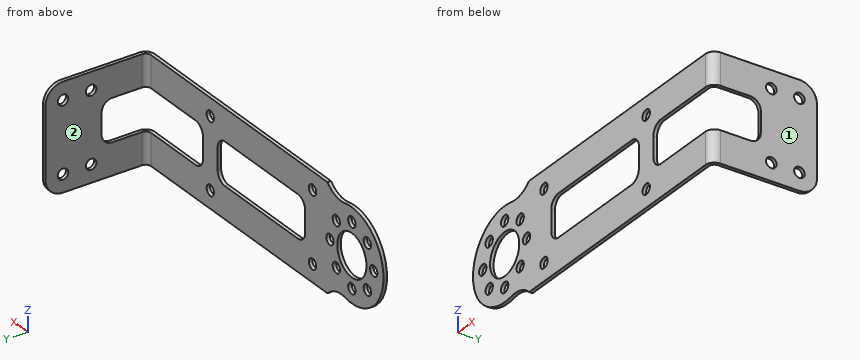
```python
from build123d import *

# Parameters (mm, degrees)
BASE_FLANGE1_DEPTH           = 1
EDGE_FLANGE1_STRIP_W         = 7
EDGE_FLANGE1_STRIP_H         = 1
EDGE_FLANGE1_STRIP_CUT_DEPTH = 30
EDGE_FLANGE1_DEPTH           = 30
FILLET1_R                    = 5
UNFOLD1_OUTLINE_W            = 3.141592654
UNFOLD1_OUTLINE_H            = 30
UNFOLD1_DEPTH                = 29
UNFOLD1_START                = -1
UNFOLD1_2_DEPTH              = 1
SKETCH10_R                   = 6
SKETCH10_R_2                 = 1.5
SKETCH10_W                   = 36
SKETCH10_H                   = 12
CUT_EXTRUDE1_DEPTH           = 10
FILLET2_R                    = 3
FOLD1_START                  = 84.74315
FOLD1_OUTLINE_W              = 1
FOLD1_OUTLINE_H              = 30
FOLD1_DEPTH                  = 28.398442654
FOLD1_START_2                = 82.5
FOLD1_2_OUTLINE_R            = 1.5
FOLD1_2_DEPTH                = 2.5
FOLD1_START_3                = -16
FOLD1_3_DEPTH                = 31


with BuildPart() as part:
    # Base-Flange1: sheet metal written as solids
    # Sketch1 → Base-Flange1 (new body)
    with BuildSketch(Plane(origin=(0, 0, 0), x_dir=(1, 0, 0), z_dir=(0, 1, 0))):
        with BuildLine():
            Line((10, -15), (85, -15))
            Line((85, -15), (85, 15))
            Line((85, 15), (10, 15))
            ThreePointArc((10, 15), (6.607674197, 12.919380101), (2.632597571, 12.730649238))
            ThreePointArc((2.632597571, 12.730649238), (-13, 0), (2.632597571, -12.730649238))
            ThreePointArc((2.632597571, -12.730649238), (6.607674197, -12.919380101), (10, -15))
        make_face()
    extrude(amount=-BASE_FLANGE1_DEPTH)

    # Edge-Flange1: sheet metal written as solids
    # Edge-Flange1 strip (on a plane across the edge) → Edge-Flange1 strip cut (cut)
    with BuildSketch(Plane(origin=(85, 0, 15), x_dir=(-1, 0, 0), z_dir=(0, 0, -1))):
        with Locations((-1, -0.5)):
            Rectangle(EDGE_FLANGE1_STRIP_W, EDGE_FLANGE1_STRIP_H)
    extrude(amount=EDGE_FLANGE1_STRIP_CUT_DEPTH, mode=Mode.SUBTRACT)

    # Edge-Flange1 section (on a plane across the edge) → Edge-Flange1 (add)
    with BuildSketch(Plane(origin=(85, 0, 15), x_dir=(-1, 0, 0), z_dir=(0, 0, -1))):
        with BuildLine():
            Line((0, 1.5), (0, 29))
            Line((0, 29), (1, 29))
            Line((1, 29), (1, 1.5))
            ThreePointArc((1, 1.5), (1.439339828, 0.439339828), (2.5, 0))
            Line((2.5, 0), (2.5, -1))
            ThreePointArc((2.5, -1), (0.732233047, -0.267766953), (0, 1.5))
        make_face()
    extrude(amount=EDGE_FLANGE1_DEPTH)

    # Fillet1
    fillet1_edges = [part.edges().sort_by_distance(p)[0] for p in [
        (84.5, 29, 15),
        (84.5, 29, -15),
    ]]
    fillet(fillet1_edges, radius=FILLET1_R)

    # Unfold1: read off the stored shape, not the designer's step
    # Unfold1 outline → Unfold1 (cut)
    with BuildSketch(Plane(origin=(0, 0, 0), x_dir=(1, 0, 0), z_dir=(0, 1, 0))):
        with Locations((84.070796327, 0)):
            Rectangle(UNFOLD1_OUTLINE_W, UNFOLD1_OUTLINE_H)
    extrude(amount=UNFOLD1_DEPTH, mode=Mode.SUBTRACT)

    # Unfold1 2 outline → Unfold1 2 (add)
    with BuildSketch(Plane(origin=(0, 0, 0), x_dir=(1, 0, 0), z_dir=(0, 1, 0)).offset(UNFOLD1_START)):
        with BuildLine():
            Line((108.141592654, 15), (82.5, 15))
            Line((82.5, 15), (82.5, -15))
            Line((82.5, -15), (108.141592654, -15))
            ThreePointArc((108.141592654, -15), (111.67712656, -13.535533906), (113.141592654, -10))
            Line((113.141592654, -10), (113.141592654, 10))
            ThreePointArc((113.141592654, 10), (111.67712656, 13.535533906), (108.141592654, 15))
        make_face()
    extrude(amount=UNFOLD1_2_DEPTH)

    # Sketch10 → Cut-Extrude1 (cut)
    with BuildSketch(Plane(origin=(0, 0, 0), x_dir=(1, 0, 0), z_dir=(0, 1, 0))):
        with Locations(Location((0, 0, 0), (0, 0, 270))):
            Circle(SKETCH10_R)
        with Locations(Location((0, 9, 0), (0, 0, 270))):
            Circle(SKETCH10_R_2)
        with Locations(Location((6.363961031, 6.363961031, 0), (0, 0, 270))):
            Circle(SKETCH10_R_2)
        with Locations(Location((9, 0, 0), (0, 0, 270))):
            Circle(SKETCH10_R_2)
        with Locations(Location((6.363961031, -6.363961031, 0), (0, 0, 270))):
            Circle(SKETCH10_R_2)
        with Locations(Location((0, -9, 0), (0, 0, 270))):
            Circle(SKETCH10_R_2)
        with Locations(Location((-6.363961031, -6.363961031, 0), (0, 0, 270))):
            Circle(SKETCH10_R_2)
        with Locations(Location((-9, 0, 0), (0, 0, 270))):
            Circle(SKETCH10_R_2)
        with Locations(Location((-6.363961031, 6.363961031, 0), (0, 0, 270))):
            Circle(SKETCH10_R_2)
        with Locations(Location((16.141592654, 10, 0), (0, 0, 270))):
            Circle(SKETCH10_R_2)
        with Locations(Location((16.141592654, -10, 0), (0, 0, 270))):
            Circle(SKETCH10_R_2)
        with Locations(Location((58.141592654, 10, 0), (0, 0, 270))):
            Circle(SKETCH10_R_2)
        with Locations(Location((58.141592654, -10, 0), (0, 0, 270))):
            Circle(SKETCH10_R_2)
        with Locations(Location((100.141592654, 10, 0), (0, 0, 270))):
            Circle(SKETCH10_R_2)
        with Locations(Location((108.141592654, 10, 0), (0, 0, 270))):
            Circle(SKETCH10_R_2)
        with Locations(Location((100.141592654, -10, 0), (0, 0, 270))):
            Circle(SKETCH10_R_2)
        with Locations(Location((108.141592654, -10, 0), (0, 0, 270))):
            Circle(SKETCH10_R_2)
        with Locations((37.141592654, 0)):
            Rectangle(SKETCH10_W, SKETCH10_H)
        with Locations((79.141592654, 0)):
            Rectangle(SKETCH10_W, SKETCH10_H)
    extrude(amount=-CUT_EXTRUDE1_DEPTH, mode=Mode.SUBTRACT)

    # Fillet2
    fillet2_edges = [part.edges().sort_by_distance(p)[0] for p in [
        (97.141592654, -0.5, -6),
        (97.141592654, -0.5, 6),
        (61.141592654, -0.5, 6),
        (61.141592654, -0.5, -6),
        (55.141592654, -0.5, -6),
        (55.141592654, -0.5, 6),
        (19.141592654, -0.5, 6),
        (19.141592654, -0.5, -6),
    ]]
    fillet(fillet2_edges, radius=FILLET2_R)

    # Fold1: read off the stored shape, not the designer's step
    # Fold1 outline → Fold1 (cut)
    with BuildSketch(Plane.YZ.offset(FOLD1_START)):
        with Locations((-0.5, 0)):
            Rectangle(FOLD1_OUTLINE_W, FOLD1_OUTLINE_H)
    extrude(amount=FOLD1_DEPTH, mode=Mode.SUBTRACT)

    # Fold1 2 outline → Fold1 2 (add)
    with BuildSketch(Plane.YZ.offset(FOLD1_START_2)):
        with BuildLine():
            Line((10, -6), (0, -6))
            Line((0, -6), (0, -15))
            Line((0, -15), (24, -15))
            ThreePointArc((24, -15), (27.535533906, -13.535533906), (29, -10))
            Line((29, -10), (29, 10))
            ThreePointArc((29, 10), (27.535533906, 13.535533906), (24, 15))
            Line((24, 15), (0, 15))
            Line((0, 15), (0, 6))
            Line((0, 6), (10, 6))
            ThreePointArc((10, 6), (12.121320344, 5.121320344), (13, 3))
            Line((13, 3), (13, -3))
            ThreePointArc((13, -3), (12.121320344, -5.121320344), (10, -6))
        make_face()
        with Locations((16, -10)):
            Circle(FOLD1_2_OUTLINE_R, mode=Mode.SUBTRACT)
        with Locations((24, -10)):
            Circle(FOLD1_2_OUTLINE_R, mode=Mode.SUBTRACT)
        with Locations((16, 10)):
            Circle(FOLD1_2_OUTLINE_R, mode=Mode.SUBTRACT)
        with Locations((24, 10)):
            Circle(FOLD1_2_OUTLINE_R, mode=Mode.SUBTRACT)
    extrude(amount=FOLD1_2_DEPTH)

    # Fold1 3 outline → Fold1 3 (cut)
    with BuildSketch(Plane.XY.offset(FOLD1_START_3)):
        with BuildLine():
            Line((84, 29), (82.5, 29))
            Line((82.5, 29), (82.5, 0))
            ThreePointArc((82.5, 0), (83.560660172, 0.439339828), (84, 1.5))
            Line((84, 1.5), (84, 29))
        make_face()
        with BuildLine():
            Line((85, 0), (85, 1.5))
            ThreePointArc((85, 1.5), (84.267766953, -0.267766953), (82.5, -1))
            Line((82.5, -1), (84.74315, -1))
            Line((84.74315, -1), (84.74315, 0))
            Line((84.74315, 0), (85, 0))
        make_face()
    extrude(amount=FOLD1_3_DEPTH, mode=Mode.SUBTRACT)


solid = part.part
```
For this review, take the finished solid that the model builds, in its own axes (mm). Face numbers are marked on the shaded views. A direction names the side the tool comes from. Round coordinates to 2 decimals unless told otherwise and drop trailing zeros. Order: outer loops, then holes, each group sorted by start corner. A loop starts at its lowest first (then second) coordinate and runs counter-clockwise, first axis right, second up. Notation, with made-up numbers: (85, 77.5) -> (139, 77.5) arc R21 cw to (139, 89.5) -> close; hole circle Ø8 at (14.25, 70). An arc over 180 degrees is marked (long way). Use a Markdown table: item, result.
Item 1: Take a section at A-A (y = 8.5). State the section outline as (x, z) points, plus the area to 3 significant figures.
Resolved:
| item | result |
|---|---|
| outline | (84, -15) -> (85, -15) -> (85, -6) -> (84, -6) -> close; (84, 6) -> (85, 6) -> (85, 15) -> (84, 15) -> close |
| area | 18.0 mm² |
Item 2: Take a section at B-B (z = 0). State the section outline as (x, y) points, plus the area to 3 significant figures.
Resolved:
| item | result |
|---|---|
| outline | (-13, -1) -> (-10.5, -1) -> (-10.5, 0) -> (-13, 0) -> close; (-7.5, -1) -> (-6, -1) -> (-6, 0) -> (-7.5, 0) -> close; (6, -1) -> (7.5, -1) -> (7.5, 0) -> (6, 0) -> close; (10.5, -1) -> (19.14, -1) -> (19.14, 0) -> (10.5, 0) -> close; (55.14, -1) -> (61.14, -1) -> (61.14, 0) -> (55.14, 0) -> close; (84, 13) -> (85, 13) -> (85, 29) -> (84, 29) -> close |
| area | 36.1 mm² |
Item 3: For pin 1 (4 mm diameter, centred on x = 58.14, z = 10, fed in from +Y); pin 2 (1.1 mm diameter, centred on y = -0.5, z = -1, fed in from +X); pin 3 (8 mm diameter, centred on y = 15.5, z = 6.5, fed in from -X), all flat-tipped, find the tip position at first contact; note any pin that passes through.
Resolved:
| item | result |
|---|---|
| pin 1 | stops at y = 0 |
| pin 2 | stops at x = 61.14 |
| pin 3 | stops at x = 84 |
Item 4: Take a section at C-C (x = 28.5). State the section outline as (y, z) points, plus the area to 3 significant figures.
Resolved:
| item | result |
|---|---|
| outline | (-1, -15) -> (0, -15) -> (0, -6) -> (-1, -6) -> close; (-1, 6) -> (0, 6) -> (0, 15) -> (-1, 15) -> close |
| area | 18.0 mm² |
Item 5: For line 1 along Y through (x, z) = (76.5, 7.5); line 2 along X through (y, z) = (-0.4, 9); line 3 along X through (y, z) = (19.25, -13), list the stretches that pass through material, from the lowest coordinate up. Write a range as [from, to].
Resolved:
| item | result |
|---|---|
| line 1 | y = [-1, 0] |
| line 2 | x = [-9.38, -1.5], [1.5, 15.02], [17.26, 57.02], [59.26, 84.12] |
| line 3 | x = [84, 85] |
Item 6: Take a section at D-D (y = 16). State the section outline as (x, z) points.
Resolved:
| item | result |
|---|---|
| outline | (84, -15) -> (85, -15) -> (85, -11.5) -> (84, -11.5) -> close; (84, -8.5) -> (85, -8.5) -> (85, 8.5) -> (84, 8.5) -> close; (84, 11.5) -> (85, 11.5) -> (85, 15) -> (84, 15) -> close |
Item 7: Machinability: for the marked faces 1 and 2, which of the approach directions +Z, -Z, +X, -X, +Y, -Y give a long, thin tool a straight path to every point of the face, cutting with its end or side? Answer none if there is none.
Resolved:
| item | result |
|---|---|
| face 1 | +Z, -Z, +X, +Y, -Y |
| face 2 | +Z, -Z, -X, +Y |
